Verification items for the finished model (mm, model axes). A direction names the side the tool comes from. Round coordinates to 2 decimals unless told otherwise and drop trailing zeros. Order: outer loops, then holes, each group sorted by start corner. A loop starts at its lowest first (then second) coordinate and runs counter-clockwise, first axis right, second up. Notation, with made-up numbers: (-28, 18) -> (4, 18) arc R26 ccw to (4, 37) -> close; hole circle Ø4 at (32.25, 10). An arc over 180 degrees is marked (long way). Answer in a Markdown table with one row per item. Add a question column.
```python
from build123d import *

# Parameters (mm, degrees)
SKETCH_W        = 200
SKETCH_H        = 200
PAD_DEPTH       = 5
SKETCH001_W     = 28.435717
SKETCH001_H     = 96.211274
SKETCH001_W_2   = 31.50908
SKETCH001_H_2   = 95.352357
PAD001_DEPTH    = 3
POCKET_DEPTH    = 5
SKETCH003_R     = 25
SKETCH003_R_2   = 15
POCKET001_DEPTH = 5
SKETCH004_R     = 8
SKETCH004_R_2   = 10
POCKET002_DEPTH = 5
PAD002_DEPTH    = 5


with BuildPart() as part:
    # Sketch → Pad (new body)
    with BuildSketch(Plane.XY):
        Rectangle(SKETCH_W, SKETCH_H)
        with BuildLine():
            ThreePointArc((-17.654241, 85), (-23.154241, 90.5), (-28.654241, 85))
            Line((-28.654241, 85), (-28.654241, 5))
            ThreePointArc((-28.654241, 5), (-23.154241, -0.5), (-17.654241, 5))
            Line((-17.654241, 5), (-17.654241, 85))
        make_face(mode=Mode.SUBTRACT)
        with BuildLine():
            ThreePointArc((30.5, 84.999994), (25, 90.499994), (19.5, 84.999994))
            Line((19.5, 5.000005), (19.5, 84.999994))
            ThreePointArc((19.5, 5.000005), (25, -0.499995), (30.5, 5.000005))
            Line((30.5, 84.999994), (30.5, 5.000005))
        make_face(mode=Mode.SUBTRACT)
    extrude(amount=PAD_DEPTH)

    # Sketch001 → Pad001 (join)
    with BuildSketch(Plane.XY):
        with Locations((-24.708835, 45.889106)):
            Rectangle(SKETCH001_W, SKETCH001_H)
        with BuildLine():
            ThreePointArc((-21.554241, 85), (-23.154241, 86.6), (-24.754241, 85))
            Line((-24.754241, 85), (-24.754241, 5))
            ThreePointArc((-24.754241, 5), (-23.154241, 3.4), (-21.554241, 5))
            Line((-21.554241, 5), (-21.554241, 85))
        make_face(mode=Mode.SUBTRACT)
        with Locations((28.35321, 45.459647)):
            Rectangle(SKETCH001_W_2, SKETCH001_H_2)
        with BuildLine():
            ThreePointArc((26.6, 85.000005), (25, 86.600005), (23.4, 85.000005))
            Line((23.4, 85.000005), (23.4, 5.000005))
            ThreePointArc((23.4, 5.000005), (25, 3.400005), (26.6, 5.000005))
            Line((26.6, 5.000005), (26.6, 85.000005))
        make_face(mode=Mode.SUBTRACT)
    extrude(amount=PAD001_DEPTH)

    # Sketch002 (on Face5 of Pad001) → Pocket (cut)
    with BuildSketch(Plane.XY.offset(5)):
        Polygon((-95, -5), (-95, -95), (-5, -95), align=None)
        Polygon((94.994808, -4.99544), (94.994808, -95.00456), (5.005192, -95.00456), align=None)
        Polygon((0, -78.141), (-72.507856, -5.633144), (72.492144, -5.633144), align=None)
    extrude(amount=-POCKET_DEPTH, mode=Mode.SUBTRACT)

    # Sketch003 (on Face5 of Pocket) → Pocket001 (cut)
    with BuildSketch(Plane.XY.offset(5)):
        with Locations((-60, 65)):
            Circle(SKETCH003_R)
        with Locations((-75, 20)):
            Circle(SKETCH003_R_2)
        with Locations((75, 20)):
            Circle(SKETCH003_R_2)
        with Locations((60, 65)):
            Circle(SKETCH003_R)
    extrude(amount=-POCKET001_DEPTH, mode=Mode.SUBTRACT)

    # Sketch004 → Pocket002 (cut)
    with BuildSketch(Plane.XY):
        with Locations((-5, 14.771259)):
            Circle(SKETCH004_R)
        with Locations((5, 29.771259)):
            Circle(SKETCH004_R)
        with Locations((-0.442374, 49.771259)):
            Circle(SKETCH004_R_2)
        with Locations((-5, 84.771259)):
            Circle(SKETCH004_R)
        with Locations((5, 69.771259)):
            Circle(SKETCH004_R)
    extrude(amount=POCKET002_DEPTH, mode=Mode.SUBTRACT)

    # Sketch005 → Pad002 (join)
    with BuildSketch(Plane.XY):
        Polygon((-97.778632, -86.74954), (-95.572601, -99.607414), (-82.526855, -99.607414), (-42.874022, -51.133889), (-57.164055, -37.100334), align=None)
        Polygon((57.164055, -37.100334), (42.874022, -51.133889), (82.526855, -99.607414), (95.572601, -99.607414), (97.778632, -86.74954), align=None)
    extrude(amount=PAD002_DEPTH)


solid = part.part
```
1) Draft check along X on faces 1 (the face through (-1, 100, 2)), 2 (the face through (-100, -1, 2)), 3 (the face through (94.995, -44, 3)). Enter one of: +X half, -X half, draft (parallel to the pull), parting line (faces both ways), or undercut.
2) Cross-section at D-D, the plane x = 68. Record the boundary of the cut face in (y, z).
3) Cross-section at A-A, the plane y = -60.5. Record the boundary of the cut face in (x, z), and give its area (3 significant figures).
4) Thickness scan on L1, parallel to Y at x = -75, z = 1.15; L2, parallel to X at y = -20.5, z = 1.35; L3, parallel to X at y = 60.5, z = 3.35. Record the ranges inside material, lowest first. Write a range as [from, to].
5) Cross-section at B-B, the plane x = -75. Record the boundary of the cut face in (y, z), and give its area (3 significant figures).
6) Cross-section at C-C, the plane y = -26. Record the boundary of the cut face in (x, z).
7) Tool access check on faces 4 (the face through (-23.3, -0.5, 4)), 5 (the face through (-25, -75, 3)). Record the directions out of +Z, -Z, +X, -X, +Y, -Y that give a thin tool (end or side, any length) a straight path to the whole face; none if there is none.
Results below:
| question | item | result |
|---|---|---|
| 1 | face 1 | draft |
| 1 | face 2 | -X half |
| 1 | face 3 | undercut |
| 2 | outline | (-100, 0) -> (-95, 0) -> (-95, 5) -> (-100, 5) -> close; (-81.85, 0) -> (-50.35, 0) -> (-50.35, 5) -> (-81.85, 5) -> close; (-32, 0) -> (-10.13, 0) -> (-10.13, 5) -> (-32, 5) -> close; (-5.63, 0) -> (6.73, 0) -> (6.73, 5) -> (-5.63, 5) -> close; (33.27, 0) -> (41.31, 0) -> (41.31, 5) -> (33.27, 5) -> close; (88.69, 0) -> (100, 0) -> (100, 5) -> (88.69, 5) -> close |
| 3 | outline | (-100, 0) -> (-95, 0) -> (-95, 5) -> (-100, 5) -> close; (-76.31, 0) -> (-50.54, 0) -> (-50.54, 5) -> (-76.31, 5) -> close; (-39.5, 0) -> (-17.64, 0) -> (-17.64, 5) -> (-39.5, 5) -> close; (17.64, 0) -> (39.5, 0) -> (39.5, 5) -> (17.64, 5) -> close; (50.54, 0) -> (76.31, 0) -> (76.31, 5) -> (50.54, 5) -> close; (94.99, 0) -> (100, 0) -> (100, 5) -> (94.99, 5) -> close |
| 3 | area | 526 mm² |
| 4 | L1 | [-100, -95], [-90.41, -58.9], [-25, 5], [35, 45], [85, 100] |
| 4 | L2 | [-100, -95], [-79.5, -57.64], [57.63, 79.49], [94.99, 100] |
| 4 | L3 | [-100, -84.59], [-35.41, -28.65], [-17.65, 19.5], [30.5, 35.41], [84.59, 100] |
| 5 | outline | (-100, 0) -> (-95, 0) -> (-95, 5) -> (-100, 5) -> close; (-90.41, 0) -> (-58.9, 0) -> (-58.9, 5) -> (-90.41, 5) -> close; (-25, 0) -> (5, 0) -> (5, 5) -> (-25, 5) -> close; (35, 0) -> (45, 0) -> (45, 5) -> (35, 5) -> close; (85, 0) -> (100, 0) -> (100, 5) -> (85, 5) -> close |
| 5 | area | 458 mm² |
| 6 | outline | (-100, 0) -> (-95, 0) -> (-95, 5) -> (-100, 5) -> close; (-74, 0) -> (-52.14, 0) -> (-52.14, 5) -> (-74, 5) -> close; (52.13, 0) -> (73.99, 0) -> (73.99, 5) -> (52.13, 5) -> close; (94.99, 0) -> (100, 0) -> (100, 5) -> (94.99, 5) -> close |
| 7 | face 4 | +Z |
| 7 | face 5 | +Z, -Z |
